from build123d import *

# Parameters (mm, degrees)
SKETCH1_R           = 82.5
BOSS_EXTRUDE1_DEPTH = 20
SKETCH2_R           = 15
CUT_EXTRUDE1_DEPTH  = 20
SKETCH3_R           = 49.5
SKETCH3_R_2         = 34.5
CUT_EXTRUDE2_DEPTH  = 9
SKETCH4_R           = 2.5
CUT_EXTRUDE3_DEPTH  = 13
SKETCH5_R           = 2
CUT_EXTRUDE4_DEPTH  = 17
SKETCH7_R           = 21.2
SKETCH7_R_2         = 15
CUT_EXTRUDE5_DEPTH  = 10
BOSS_EXTRUDE2_DEPTH = 3


with BuildPart() as part:
    # Sketch1 → Boss-Extrude1 (new body)
    with BuildSketch(Plane(origin=(0, 0, 0), x_dir=(1, 0, 0), z_dir=(0, 1, 0))):
        Circle(SKETCH1_R)
    extrude(amount=BOSS_EXTRUDE1_DEPTH)

    # Sketch2 → Cut-Extrude1 (cut)
    with BuildSketch(Plane(origin=(0, 20, 0), x_dir=(1, 0, 0), z_dir=(0, 1, 0))):
        Circle(SKETCH2_R)
    extrude(amount=-CUT_EXTRUDE1_DEPTH, mode=Mode.SUBTRACT)

    # Sketch3 → Cut-Extrude2 (cut)
    with BuildSketch(Plane(origin=(0, 20, 0), x_dir=(1, 0, 0), z_dir=(0, 1, 0))):
        Circle(SKETCH3_R)
        Circle(SKETCH3_R_2, mode=Mode.SUBTRACT)
    extrude(amount=-CUT_EXTRUDE2_DEPTH, mode=Mode.SUBTRACT)

    # Sketch4 → Cut-Extrude3 (cut)
    with BuildSketch(Plane.XZ):
        with Locations((0, 70)):
            Circle(SKETCH4_R)
        with Locations((60.621778265, 35)):
            Circle(SKETCH4_R)
        with Locations((60.621778265, -35)):
            Circle(SKETCH4_R)
        with Locations((0, -70)):
            Circle(SKETCH4_R)
        with Locations((-60.621778265, -35)):
            Circle(SKETCH4_R)
        with Locations((-60.621778265, 35)):
            Circle(SKETCH4_R)
    extrude(amount=-CUT_EXTRUDE3_DEPTH, mode=Mode.SUBTRACT)

    # Sketch5 → Cut-Extrude4 (cut)
    with BuildSketch(Plane.XZ):
        with Locations((31.819805153, 31.819805153)):
            Circle(SKETCH5_R)
        with Locations((31.819805153, -31.819805153)):
            Circle(SKETCH5_R)
        with Locations((-31.819805153, -31.819805153)):
            Circle(SKETCH5_R)
        with Locations((-31.819805153, 31.819805153)):
            Circle(SKETCH5_R)
    extrude(amount=-CUT_EXTRUDE4_DEPTH, mode=Mode.SUBTRACT)

    # Sketch7 → Cut-Extrude5 (cut)
    with BuildSketch(Plane(origin=(0, 20, 0), x_dir=(1, 0, 0), z_dir=(0, 1, 0))):
        Circle(SKETCH7_R)
        Circle(SKETCH7_R_2, mode=Mode.SUBTRACT)
    extrude(amount=-CUT_EXTRUDE5_DEPTH, mode=Mode.SUBTRACT)

    # Sketch8 → Boss-Extrude2 (add)
    with BuildSketch(Plane(origin=(0, 20, 0), x_dir=(1, 0, 0), z_dir=(0, 1, 0))):
        with BuildLine():
            Line((-5, 82.34834546), (-5, 76.84834546))
            Line((-5, 76.84834546), (-3, 76.84834546))
            Line((-3, 76.84834546), (-3, 82.445436502))
            ThreePointArc((-3, 82.445436502), (-4.000294573, 82.402958948), (-5, 82.34834546))
        make_face()
        with BuildLine():
            Line((5, 76.84834546), (5, 82.34834546))
            ThreePointArc((5, 82.34834546), (4.000294573, 82.402958948), (3, 82.445436502))
            Line((3, 82.445436502), (3, 76.84834546))
            Line((3, 76.84834546), (5, 76.84834546))
        make_face()
        with BuildLine():
            Line((64.052619407, 42.754299749), (65.052619407, 41.022248941))
            Line((65.052619407, 41.022248941), (69.899842437, 43.820794462))
            ThreePointArc((69.899842437, 43.820794462), (69.362908509, 44.665836196), (68.815759128, 45.504299749))
            Line((68.815759128, 45.504299749), (64.052619407, 42.754299749))
        make_face()
        with BuildLine():
            Line((69.052619407, 34.094045711), (73.815759128, 36.844045711))
            ThreePointArc((73.815759128, 36.844045711), (73.363203082, 37.737122751), (72.899842437, 38.62464204))
            Line((72.899842437, 38.62464204), (68.052619407, 35.826096519))
            Line((68.052619407, 35.826096519), (69.052619407, 34.094045711))
        make_face()
        with BuildLine():
            Line((-64.052619407, 42.754299749), (-68.815759128, 45.504299749))
            ThreePointArc((-68.815759128, 45.504299749), (-69.362908509, 44.665836196), (-69.899842437, 43.820794462))
            Line((-69.899842437, 43.820794462), (-65.052619407, 41.022248941))
            Line((-65.052619407, 41.022248941), (-64.052619407, 42.754299749))
        make_face()
        with BuildLine():
            Line((-69.052619407, 34.094045711), (-73.815759128, 36.844045711))
            ThreePointArc((-73.815759128, 36.844045711), (-73.363203082, 37.737122751), (-72.899842437, 38.62464204))
            Line((-72.899842437, 38.62464204), (-68.052619407, 35.826096519))
            Line((-68.052619407, 35.826096519), (-69.052619407, 34.094045711))
        make_face()
    extrude(amount=BOSS_EXTRUDE2_DEPTH)


solid = part.part
The listing builds one solid part. Answer for the finished solid, in the listing's coordinates (mm). A direction names the side the tool comes from. Give positions to 0.01 mm unless a question says otherwise; leave off trailing zeros. Write each loop counter-clockwise with the first axis right and the second up, starting at its lowest first coordinate (ties: lowest second). Pieces come first, ordered by that corner, then holes.
1) Given P1, Ø12, axis at y = 5.5, z = -19.5, coming from the +X side; P2, Ø1.5, axis at x = 47.5, z = -34.5, coming from the -Y side; P3, Ø4, axis at y = 6.5, z = -30, coming from the +X side; P4, Ø2, axis at x = -19.5, y = 8.5, coming from the -Z side, each flat-ended and moving along its own axis, determine where each tip first touches the part or whether it passes through.
2) Find the intervals of material crossed by L1, parallel to X at y = 14, z = 0; L2, parallel to Z at x = -29, y = 11.5, in increasing order.
3) For a pull along Z with two mould halves and no side action, classify faces 1 (the face through (-61, 13, 35)), 2 (the face through (67, 23, -43)), 3 (the face through (-5, 10, -14.4)) as pulls with the +Z half, pulls with the -Z half, needs draft (parallel to the pull), parting line crosses it, or undercut.
4) Section D-D (z = 70) is taken. Write down the section's boundary in (x, y).
5) Section B-B (y = 18) is taken. Write down the section's boundary in (x, z), and give its area (3 significant figures).
6) A tool of negligible diameter and unlimited length cuts with its end or side. For faces 4 (the face through (-14.985, 5.07, -0.66)), 5 (the face through (19.583, 15.07, 8.12)), 6 (the face through (-61, 13, -35)), from which of +Z, -Z, +X, -X, +Y, -Y can it reach the whole face along a straight path? Write none if from no direction.
7) Section A-A (z = 0) is taken. Write down the section's boundary in (x, y), and give its area (3 significant figures).
8) Section C-C (x = 12) is taken. Write down the section's boundary in (y, z), and give its area (3 significant figures).
Response:
1. P1: stops at x = 81.39
1. P2: stops at y = 0
1. P3: stops at x = 77.6
1. P4: stops at z = -80.4
2. L1: x = -82.5 to -49.5, -34.5 to -21.2, 21.2 to 34.5, 49.5 to 82.5
2. L2: z = -77.24 to -40.12, -18.69 to 18.69, 40.12 to 77.24
3. face 1: undercut
3. face 2: needs draft
3. face 3: undercut
4. outline: (-43.66, 0) - (-2.5, 0) - (-2.5, 13) - (2.5, 13) - (2.5, 0) - (43.66, 0) - (43.66, 20) - (-43.66, 20) - close
5. outline: circle Ø165 at (0, 0); circle Ø69 at (0, 0); hole circle Ø99 at (0, 0); hole circle Ø42.4 at (0, 0)
5. area: 16,000 mm2
6. face 4: +Y, -Y
6. face 5: +Y
6. face 6: -Y
7. outline: (-82.5, 0) - (-15, 0) - (-15, 10) - (-21.2, 10) - (-21.2, 20) - (-34.5, 20) - (-34.5, 11) - (-49.5, 11) - (-49.5, 20) - (-82.5, 20) - close; (15, 0) - (82.5, 0) - (82.5, 20) - (49.5, 20) - (49.5, 11) - (34.5, 11) - (34.5, 20) - (21.2, 20) - (21.2, 10) - (15, 10) - close
7. area: 2,310 mm2
8. outline: (0, -81.62) - (20, -81.62) - (20, -48.02) - (11, -48.02) - (11, -32.35) - (20, -32.35) - (20, -17.48) - (10, -17.48) - (10, -9) - (0, -9) - close; (0, 9) - (10, 9) - (10, 17.48) - (20, 17.48) - (20, 32.35) - (11, 32.35) - (11, 48.02) - (20, 48.02) - (20, 81.62) - (0, 81.62) - close
8. area: 2,450 mm2
